Can you work these out from the model? Positions are in its coordinate system, mm. Give positions to 0.01 mm unless a question says otherwise; leave off trailing zeros. Loops run counter-clockwise (first coordinate to the right, second up) from the corner with the lowest first, then second, coordinate; pieces in that order, holes last. Notation, with made-up numbers: (65, 31.25) -> (95, 31.25) arc R24 ccw to (95, 41.25) -> close; hole circle Ø1 at (32, -30). An arc over 180 degrees is marked (long way). Use CSV: the item, a comma, the result in double quotes.
Autodesk Inventor part; units mm, degrees
ref_plane "YZ Plane" through (0, 0, 0) normal (1, 0, 0) x (0, 1, 0)
ref_plane "XZ Plane" through (0, 0, 0) normal (0, 1, 0) x (-1, 0, 0)
ref_plane "XY Plane" through (0, 0, 0) normal (0, 0, 1) x (1, 0, 0)
sketch "Sketch1" plane through (0, 0, 0) normal (0, 0, 1) x (1, 0, 0)
  circle A0 centre (0, 0) radius 4.5
  dimension "d0" = 9
extrude "Extrusion1" add sketch "Sketch1" along normal blind 100
sketch "Sketch2" plane through (0, 0, 0) normal (1, 0, 0) x (0, 1, 0)
  line L0 (0, 0) -> (0, 1)
  line L1 (0, 0) -> (0, 6.35)
  line L2 (0, 0) -> (-10, 0)
  line L3 (-4.5, 0) -> (4.5, 0)
  line L4 (0, 0) -> (0, 9.525)
  line L5 (0, 9.525) -> (0, 0)
  line L6 (0, 0) -> (0, 10)
  circle A0 centre (0, 10) radius 1
  dimension "d3" = 1
  dimension "d4" = 10
  dimension "d5" = 10
  dimension "d6" = 2
extrude "Extrusion2" cut sketch "Sketch2" along normal through all both and the other way through all
thread "Thread1"
properties part number "1"
(1) Will this pin go through, and if not, where does the flat tip stop? pin 1 Ø1.5 at (x, z) = (1, 45) entering from -Y.
Answer sheet:
pin 1,"stops at y = -4.49"
(2) If we section it at D-D, the plane y = 3: Write out the boundary of the cut face in (x, z).
Answer sheet:
outline,"(-3.35, 0) -> (3.35, 0) -> (3.35, 100) -> (-3.35, 100) -> close"
(3) If we section it at A-A, the plane z = 10: Write out the boundary of the cut face in (x, y).
Answer sheet:
outline,"(-4.39, -1) arc R4.5 ccw to (4.39, -1) -> close; (-4.39, 1) -> (4.39, 1) arc R4.5 ccw to start"
(4) If we section it at B-B, the plane x = -1.75: Write out the boundary of the cut face in (y, z), then the cut area to 3 significant figures.
Answer sheet:
outline,"(-4.15, 0) -> (4.15, 0) -> (4.15, 100) -> (-4.15, 100) -> close; hole circle Ø2 at (0, 10)"
area,"826 mm2"
(5) If I drill on L1, parallel to Y at x = 0, z = 10; L2, parallel to Z at x = 0.5, y = 0; L3, parallel to Y at x = 2, z = 10, over which ranges is the centre line in solid material (lowest first)? Write a range as from..to.
Answer sheet:
L1,"y = -4.5..-1, 1..4.5"
L2,"z = 0..9, 11..100"
L3,"y = -4.03..-1, 1..4.03"
(6) We'd pull the mould along Z, two halves only. Please class faces 1 (the face through (0, 0, 0)), 2 (the face through (4.16, 1.72, 49.3)), 3 (the face through (0, 0, 9)), 4 (the face through (0, 0, 100)): released by +Z, released by -Z, zero draft, split by the parting line, or undercut.
Answer sheet:
face 1,"released by -Z"
face 2,"zero draft"
face 3,"undercut"
face 4,"released by +Z"
(7) If we section it at C-C, the plane z = 79: Write out the boundary of the cut face in (x, y), then the cut area to 3 significant figures.
Answer sheet:
outline,"circle Ø9 at (0, 0)"
area,"63.6 mm2"
